from build123d import *

# Parameters (mm, degrees)
BOSS_EXTRUDE1_DEPTH = 450
FILLET1_R           = 13.4
BOSS_EXTRUDE2_DEPTH = 450
FILLET2_R           = 13.4
CUT_EXTRUDE1_DEPTH  = 451.0000001
SHELL1_T            = -1
BOSS_EXTRUDE3_DEPTH = 450
CUT_EXTRUDE2_DEPTH  = 13.698698186


with BuildPart() as part:
    # Sketch2 → Boss-Extrude1 (new body)
    with BuildSketch(Plane.XY):
        Polygon((0, 0), (151.490860479, 0), (151.490860479, 23.2), (1.215860479, 23.2), align=None)
    extrude(amount=BOSS_EXTRUDE1_DEPTH)

    # Fillet1
    fillet1_edges = [part.edges().sort_by_distance(p)[0] for p in [
        (1.215860479, 23.2, 225),
    ]]
    fillet(fillet1_edges, radius=FILLET1_R)

    # Sketch4 → Boss-Extrude2 (add, through all)
    with BuildSketch(Plane.XY.offset(450)):
        with BuildLine():
            Line((24.166834741, -1.266530141), (23.567700201, -12.698698186))
            ThreePointArc((23.567700201, -12.698698186), (27.725384653, -3.679983428), (36.949335967, 0))
            Line((36.949335967, 0), (0, 0))
            Line((0, 0), (9.586843534, -0.50242518))
            Line((9.586843534, -0.50242518), (9.22049184, -7.492831923))
            Line((9.22049184, -7.492831923), (14.213639514, -7.754511704))
            Line((14.213639514, -7.754511704), (14.579991207, -0.764104961))
            Line((14.579991207, -0.764104961), (24.166834741, -1.266530141))
        make_face()
    extrude(amount=-BOSS_EXTRUDE2_DEPTH)

    # Fillet2
    fillet2_edges = [part.edges().sort_by_distance(p)[0] for p in [
        (27.725384653, -3.679983428, 0),
        (27.725384653, -3.679983428, 450),
        (94.220098223, 0, 450),
        (94.220098223, 0, 0),
    ]]
    fillet(fillet2_edges, radius=FILLET2_R)

    # Sketch5 → Cut-Extrude1 (cut, through all)
    with BuildSketch(Plane.XY):
        with BuildLine():
            Line((24.166834741, -1.266530141), (23.567700201, -12.698698186))
            ThreePointArc((23.567700201, -12.698698186), (27.725384653, -3.679983428), (36.949335967, 0))
            Line((36.949335967, 0), (0, 0))
            Line((0, 0), (9.586843534, -0.50242518))
            Line((9.586843534, -0.50242518), (9.22049184, -7.492831923))
            Line((9.22049184, -7.492831923), (14.213639514, -7.754511704))
            Line((14.213639514, -7.754511704), (14.579991207, -0.764104961))
            Line((14.579991207, -0.764104961), (24.166834741, -1.266530141))
        make_face()
    extrude(amount=CUT_EXTRUDE1_DEPTH, mode=Mode.SUBTRACT)

    # Shell1
    shell1_openings = [part.faces().sort_by_distance(p)[0] for p in [
        (151.490860479, 11.274923044, 225),
    ]]
    offset(amount=SHELL1_T, openings=shell1_openings)

    # Sketch6 → Boss-Extrude3 (add)
    with BuildSketch(Plane.XY):
        with BuildLine():
            Line((24.166834741, -1.266530141), (23.567700201, -12.698698186))
            ThreePointArc((23.567700201, -12.698698186), (27.725384653, -3.679983428), (36.949335967, 0))
            Line((36.949335967, 0), (0, 0))
            Line((0, 0), (9.586843534, -0.50242518))
            Line((9.586843534, -0.50242518), (9.22049184, -7.492831923))
            Line((9.22049184, -7.492831923), (14.213639514, -7.754511704))
            Line((14.213639514, -7.754511704), (14.579991207, -0.764104961))
            Line((14.579991207, -0.764104961), (24.166834741, -1.266530141))
        make_face()
    extrude(amount=BOSS_EXTRUDE3_DEPTH)

    # Sketch7 → Cut-Extrude2 (cut, through all)
    with BuildSketch(Plane.XZ):
        with BuildLine():
            Line((13.739855146, 450), (36.949335967, 450))
            Line((36.949335967, 450), (36.949335967, 436.6))
            add(Edge.make_bspline(
                [(13.739855146, 450), (14.897031698, 450), (16.037346218, 449.888583323), (17.726143963, 449.5782461), (18.285436938, 449.450751492), (19.397111441, 449.150094553), (19.951343846, 448.976153087), (22.667401959, 448.011694289), (24.688899416, 446.937288096), (27.088419743, 445.339458648), (27.560915156, 445.007570641), (28.487586558, 444.326213533), (28.942650844, 443.976156414), (30.286745236, 442.902062513), (31.15469064, 442.154118787), (32.853186658, 440.615831161), (33.683710559, 439.825456971), (35.32594722, 438.223379533), (36.139219776, 437.410115889), (36.949335967, 436.6)],
                knots=[0, 0, 0, 0, 0.125, 0.125, 0.1875, 0.1875, 0.25, 0.25, 0.5, 0.5, 0.5625, 0.5625, 0.625, 0.625, 0.75, 0.75, 0.875, 0.875, 1, 1, 1, 1], degree=3))
        make_face()
        with BuildLine():
            Line((36.949335967, 13.4), (36.949335967, 0))
            Line((36.949335967, 0), (13.739855146, 0))
            add(Edge.make_bspline(
                [(36.949335967, 13.4), (36.139219776, 12.589884111), (35.32594722, 11.776620467), (33.683710559, 10.174543029), (32.853186658, 9.384168839), (31.15469064, 7.845881213), (30.286745236, 7.097937487), (28.942650844, 6.023843586), (28.487586558, 5.673786467), (27.560915156, 4.992429359), (27.088419743, 4.660541352), (24.688899416, 3.062711904), (22.667401959, 1.988305711), (19.951343846, 1.023846913), (19.397111441, 0.849905447), (18.285436938, 0.549248508), (17.726143963, 0.4217539), (16.037346218, 0.111416677), (14.897031698, 0), (13.739855146, 0)],
                knots=[0, 0, 0, 0, 0.125, 0.125, 0.25, 0.25, 0.375, 0.375, 0.4375, 0.4375, 0.5, 0.5, 0.75, 0.75, 0.8125, 0.8125, 0.875, 0.875, 1, 1, 1, 1], degree=3))
        make_face()
    extrude(amount=CUT_EXTRUDE2_DEPTH, mode=Mode.SUBTRACT)


solid = part.part
Read the model definition and answer for the solid it produces. Units are mm, in the model's axes. A direction names the side the tool comes from. Give positions to 0.01 mm unless a question says otherwise; leave off trailing zeros. Write each loop counter-clockwise with the first axis right and the second up, starting at its lowest first coordinate (ties: lowest second). Pieces come first, ordered by that corner, then holes. Notation, with made-up numbers: (64.25, 43.5) - (81.25, 43.5) arc R14 ccw to (81.25, 69.5) - close; hole circle Ø10 at (4, 15.5). An arc over 180 degrees is marked (long way). Answer in a Markdown table with one row per item. Add a question column.
Item 1: Section A-A, the plane x = 133.5 is taken. Write down the section's boundary in (y, z).
Item 2: A tool of negligible diameter and unlimited length cuts with its end or side. For faces 4 (the face through (75, 16, 1)), 5 (the face through (84, 22.2, 222)), 6 (the face through (95.02, 3.82, 445.97)), from which of +Z, -Z, +X, -X, +Y, -Y can it reach the whole face along a straight path? Write none if from no direction.
Item 3: Flat-ended cylindrical pins translate along their axes: P1, Ø1.5, axis at y = 9.5, z = 290.5, coming from the +X side; P2, Ø5, axis at y = 11.5, z = 81.5, coming from the -X side; P3, Ø6, axis at x = 118.5, z = 99, coming from the -Y side. Find the tip coordinate at first contact, or state that the pin passes through.
Item 4: Section B-B, the plane z = 366 is taken. Write down the section's boundary in (x, y).
Item 5: Determine the mould class of faces 1 (the face through (19.31, -1.01, 221.85)), 2 (the face through (151.491, 23, 224)), 3 (the face through (95.02, 3.82, 4.03)) for opening direction X: pulls with the +X half, pulls with the -X half, needs draft (parallel to the pull), parting line crosses it, or undercut.
Item 6: Find the intervals of material crossed by L1, parallel to Y at x = 116, z = 174.5; L2, parallel to X at y = 2, z = 339; L3, parallel to Z at x = 132, y = 18.5, in increasing order.
Recorded:
| question | item | result |
|---|---|---|
| 1 | outline | (0, 13.4) arc R13.4 ccw to (13.4, 0) - (23.2, 0) - (23.2, 450) - (13.4, 450) arc R13.4 ccw to (0, 436.6) - close; hole (1, 13.4) arc R12.4 ccw to (13.4, 1) - (22.2, 1) - (22.2, 449) - (13.4, 449) arc R12.4 ccw to (1, 436.6) - close |
| 2 | face 4 | none |
| 2 | face 5 | +X |
| 2 | face 6 | +Z, +X, -Y |
| 3 | P1 | stops at x = 1.54 |
| 3 | P2 | stops at x = 0.47 |
| 3 | P3 | stops at y = 0 |
| 4 | outline | (0, 0) - (9.59, -0.5) - (9.22, -7.49) - (14.21, -7.75) - (14.58, -0.76) - (24.17, -1.27) - (23.57, -12.7) arc R13.4 cw to (36.95, 0) - (151.49, 0) - (151.49, 1) - (1.05, 1) - (1.55, 10.45) arc R12.4 cw to (13.93, 22.2) - (151.49, 22.2) - (151.49, 23.2) - (13.93, 23.2) arc R13.4 ccw to (0.55, 10.5) - close |
| 5 | face 1 | undercut |
| 5 | face 2 | pulls with the +X half |
| 5 | face 3 | needs draft |
| 6 | L1 | y = 0 to 1, 22.2 to 23.2 |
| 6 | L2 | x = 0.1 to 1.11 |
| 6 | L3 | z = 0 to 1, 449 to 450 |
